Check sheet for the modelled part. Datum: model origin and axes. Units: mm. Face numbers are marked on the shaded views. A direction names the side the tool comes from. Round coordinates to 2 decimals unless told otherwise and drop trailing zeros. Loops run counter-clockwise (first coordinate to the right, second up) from the corner with the lowest first, then second, coordinate; pieces in that order, holes last. Notation, with made-up numbers: (54.25, 9) -> (72.25, 9) arc R27 cw to (72.25, 30) -> close; hole circle Ø6 at (88.25, -23). An arc over 180 degrees is marked (long way). Use one line per item in the form item = value. Start each with the question number.
(1) Sectioned sample at A-A (z = 7). Record the cut outline in (x, y).
(2) Sectioned sample at B-B (y = -9). Record the cut outline in (x, z).
(3) Sectioned sample at D-D (x = 1). State how many separate pieces and enclosed holes the cut face has, and give its area (3 significant figures).
(4) Material ranges on probe 1 along Z at (x, y) = (5, 6); probe 2 along Z at (x, y) = (4.75, -1); probe 3 along X at (y, z) = (-10.5, -8.5), recorded low to high. Write a range as [from, to].
(5) Set-up check for the marked faces 5 and 6: record each of +Z, -Z, +X, -X, +Y, -Y from which the full face is reachable in a straight line by a thin tool's end or side.
(6) Sectioned sample at C-C (z = -5). Record the cut outline in (x, y).
(7) Draft check along Y on the marked faces 1, 2, 3 and 4. Enter one of: released by +Y, released by -Y, zero draft, split by the parting line, or undercut.
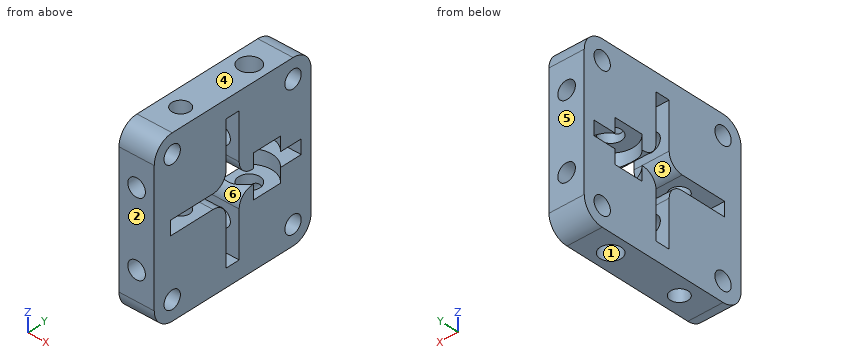
Autodesk Inventor part; units mm, degrees
ref_plane "YZ Plane" through (0, 0, 0) normal (1, 0, 0) x (0, 1, 0)
ref_plane "XZ Plane" through (0, 0, 0) normal (0, 1, 0) x (-1, 0, 0)
ref_plane "XY Plane" through (0, 0, 0) normal (0, 0, 1) x (1, 0, 0)
sketch "Sketch1" plane through (0, 0, 0) normal (1, 0, 0) x (0, 1, 0)
  circle A0 centre (0, 0) radius 2.8284
  line L0 (0, 0) -> (-2.8284, 0)
  line L1 (-2.8284, 0) -> (-2.8284, -2.8284)
  line L2 (-2.8284, -2.8284) -> (0, -2.8284)
  line L3 (0, -2.8284) -> (0, 0)
  line L4 (0, 0) -> (-2.8284, -2.8284)
  line L5 (2, 2) -> (-2, 2)
  line L6 (-2, 2) -> (-2, -2)
  line L7 (-2, -2) -> (2, -2)
  line L8 (2, -2) -> (2, 2)
  line L9 (2, 2) -> (-2, -2) construction
  line L10 (-2, 2) -> (2, -2) construction
  line L11 (2, 2) -> (-2, 2)
  line L12 (-2, 2) -> (-2, 4)
  line L13 (-2, 4) -> (2, 4)
  line L14 (2, 4) -> (2, 2)
  line L15 (0, 4) -> (0, 19)
  line L16 (-2, 2) -> (-4, 2)
  line L17 (-4, 2) -> (-4, -2)
  line L18 (-4, -2) -> (-2, -2)
  line L19 (-4, 0) -> (-19, 0)
  line L20 (19, -19) -> (19, 19)
  line L21 (19, 19) -> (-19, 19)
  line L22 (-19, 19) -> (-19, -19)
  line L23 (-19, -19) -> (19, -19)
  line L24 (19, -19) -> (-19, 19) construction
  line L25 (19, 19) -> (-19, -19) construction
  line L26 (0, 19) -> (0, 24)
  line L27 (-19, 0) -> (-24, 0)
  line L28 (24, -24) -> (24, 24)
  line L29 (24, 24) -> (-24, 24)
  line L30 (-24, 24) -> (-24, -24)
  line L31 (-24, -24) -> (24, -24)
  line L32 (24, -24) -> (-24, 24) construction
  line L33 (24, 24) -> (-24, -24) construction
  line L34 (-2, 2) -> (-19, 2)
  line L35 (-19, -2) -> (-2, -2)
  line L36 (-2, -2) -> (-2, 2)
  line L37 (-2, -2) -> (-19, -2)
  line L38 (-19, -2) -> (-19, -19)
  line L39 (-19, -19) -> (-2, -19)
  line L40 (-2, -19) -> (-2, -2)
  line L41 (2, -2) -> (19, -2)
  line L42 (19, -2) -> (19, -19)
  line L43 (19, -19) -> (2, -19)
  line L44 (2, -19) -> (2, -2)
  line L45 (2, 2) -> (19, 2)
  line L46 (19, 2) -> (19, 19)
  line L47 (19, 19) -> (2, 19)
  line L48 (2, 19) -> (2, 2)
  line L49 (-2, 2) -> (-19, 2)
  line L50 (-19, 2) -> (-19, 19)
  line L51 (-19, 19) -> (-2, 19)
  line L52 (-2, 19) -> (-2, 2)
  point P0 (-2, 19)
  point P1 (2, 4)
  point P2 (2, -19)
  point P3 (-2, -19)
  dimension "d0" = 4
  dimension "d1" = 2
  dimension "d5" = 15
  dimension "d6" = 2
  dimension "d7" = 15
  dimension "d8" = 2
  dimension "d9" = 0
  dimension "d10" = 5
  dimension "d11" = 5
  dimension "d12" = 15
  dimension "d13" = 22.6716
  dimension "d14" = 20
  dimension "d15" = 29.7321
extrude "Extrusion1" add sketch "Sketch1" along normal blind 10 contours L14 L48 L21 L20 L45 | L41 L20 L23 L44 | L16 L34 L22 L21 L52 L12 | L20 L21 L26 L29 L28 L31 L30 L27 L22 L23 | L40 L2 L4 | L4 L1 L18 | L40 L23 L22 L35 L18 L1 L2 | L21 L22 L27 L30 L29 L26
sketch "Sketch2" plane through (0, 24, 24) normal (0, 1, 0) x (1, 0, 0)
  line L0 (10, 0) -> (0, 0)
  line L1 (0, 0) -> (0, 48)
  line L2 (0, 48) -> (10, 48)
  line L3 (10, 48) -> (10, 0)
  line L4 (0, 48) -> (10, 48)
  line L5 (0, 48) -> (0, 34.5)
  line L6 (0, 34.5) -> (5, 34.5)
  circle A0 centre (5, 34.5) radius 2.5
  line L7 (0, 0) -> (0, 13.5)
  line L8 (0, 22) -> (0, 5)
  line L9 (0, 13.5) -> (5, 13.5)
  circle A1 centre (5, 13.5) radius 2.5
  point P0 (0, 24)
  dimension "d18" = 13.5
  dimension "d19" = 5
  dimension "d20" = 5
  dimension "d21" = 13.5
  dimension "d22" = 5
  dimension "d23" = 5
extrude "Extrusion2" cut sketch "Sketch2" against normal through all contours A0 | A1
sketch "Sketch3" plane through (0, -24, -24) normal (0, 0, -1) x (-1, 0, 0)
  line L0 (0, 0) -> (-10, 0)
  line L1 (0, 0) -> (0, 13.5)
  line L2 (0, 22) -> (0, 5)
  line L3 (0, 48) -> (-10, 48)
  line L4 (0, 48) -> (0, 34.5)
  line L5 (0, 0) -> (0, 48)
  line L6 (0, 34.5) -> (-5, 34.5)
  line L7 (0, 13.5) -> (-5, 13.5)
  circle A0 centre (-5, 13.5) radius 2.5
  circle A1 centre (-5, 34.5) radius 2.5
  point P0 (0, 24)
  dimension "d26" = 13.5
  dimension "d27" = 13.5
  dimension "d28" = 5
  dimension "d29" = 5
  dimension "d30" = 5
  dimension "d31" = 5
extrude "Extrusion3" cut sketch "Sketch3" against normal through all
fillet "Fillet1" radius 4 4 edges at (5, -2, 2) (5, 2, 2) (5, 2, -2) (5, -2, -2)
sketch "Sketch4" plane through (10, 0, 0) normal (1, 0, 0) x (0, 0, -1)
  line L0 (24, 24) -> (-24, 24)
  line L1 (24, 24) -> (18.5, 24)
  line L2 (18.5, 24) -> (18.5, 18.5)
  line L3 (18.5, 18.5) -> (24, 18.5)
  line L4 (24, 18.5) -> (24, 24)
  circle A0 centre (18.5, 18.5) radius 2.5
  circle A1 centre (18.5, 18.5) radius 5.5
  circle A2 centre (-18.5, 18.5) radius 5.5
  circle A3 centre (-18.5, 18.5) radius 2.5
  line L5 (-18.5, 24) -> (-24, 24)
  line L6 (-24, 24) -> (-24, 18.5)
  circle A4 centre (-18.5, -18.5) radius 5.5
  circle A5 centre (-18.5, -18.5) radius 2.5
  line L7 (-24, -18.5) -> (-24, -24)
  line L8 (-24, -24) -> (-18.5, -24)
  circle A6 centre (18.5, -18.5) radius 5.5
  circle A7 centre (18.5, -18.5) radius 2.5
  line L9 (18.5, -24) -> (24, -24)
  line L10 (24, -24) -> (24, -18.5)
  point P0 (0, 0)
  point P1 (-18.5, 24)
  dimension "d35" = 5.5
  dimension "d36" = 5.5
  dimension "d37" = 5
  dimension "d40" = 360
extrude "Extrusion4" cut sketch "Sketch4" against normal through all contours L4 A1 L0 | A2 L6 L0 | A0 L3 L2 | L2 L3 A0 | A3 | A4 L8 L7 | A5 | L10 L9 A6 | A7
sketch "Sketch5" plane through (0, -18.5, 24) normal (0, 0, 1) x (1, 0, 0)
  circle A0 centre (5, 29) radius 2.5
  circle A1 centre (5, 29) radius 3
  point P0 (0, 18.5)
  dimension "d44" = 6
extrude "Extrusion5" cut sketch "Sketch5" against normal through all contours A0 | A1
sketch "Sketch6" plane through (0, 19, -2) normal (0, 0, 1) x (1, 0, 0)
  circle A0 centre (5, -8.5) radius 6.5
  point P0 (0, -19)
extrude "Extrusion6" cut sketch "Sketch6" against normal blind 4
sketch "Sketch7" plane through (10, 19, 2) normal (0, 0, -1) x (-1, 0, 0)
  circle A0 centre (5, -8.5) radius 6.5
  point P0 (10, -19)
extrude "Extrusion7" cut sketch "Sketch7" against normal blind 4
sketch "Sketch8" plane through (10, 0, 0) normal (1, 0, 0) x (0, 0, -1)
  line L0 (-2, 14.6533) -> (-2, 19)
  line L1 (-2, 19) -> (2, 19)
  line L2 (2, 19) -> (2, 21)
  line L3 (2, 21) -> (-2, 21)
  line L4 (-2, 21) -> (-2, 19)
  point P0 (0, 0)
  dimension "d51" = 2
extrude "Extrusion8" cut sketch "Sketch8" against normal through all
properties part number "guidance_block" material "PET Plastic"
Checks:
q1.outline = (0, -24) -> (10, -24) -> (10, -2) -> (0, -2) -> close; (0, 2) -> (10, 2) -> (10, 24) -> (0, 24) -> close; hole circle Ø6 at (5, 10.5); hole circle Ø5 at (5, -10.5)
q2.outline = (0, -24) -> (3, -24) -> (3, -12) arc R2.5 cw to (3, -9) -> (3, -2) -> (0, -2) -> close; (0, 2) -> (3, 2) -> (3, 9) arc R2.5 cw to (3, 12) -> (3, 24) -> (0, 24) -> close; (7, -24) -> (10, -24) -> (10, -2) -> (7, -2) -> (7, -9) arc R2.5 cw to (7, -12) -> close; (7, 2) -> (10, 2) -> (10, 24) -> (7, 24) -> (7, 12) arc R2.5 cw to (7, 9) -> close
q3.separate_pieces = 1
q3.enclosed_holes = 5
q3.area = 1,810 mm2
q4.probe_1 = [-24, -13], [-8, -6], [6, 8], [13, 24]
q4.probe_2 = [-24, -19], [19, 24]
q4.probe_3 = [0, 2.5], [7.5, 10]
q5.face_5 = +Z, -Z, +X, -X, +Y
q5.face_6 = +X, -X
q6.outline = (0, -24) -> (10, -24) -> (10, -2.13) -> (0, -2.13) -> close; (0, 2.13) -> (10, 2.13) -> (10, 6.35) arc R6.5 cw to (0, 6.35) -> close; (0, 14.65) arc R6.5 cw to (10, 14.65) -> (10, 24) -> (0, 24) -> close; hole circle Ø5 at (5, -10.5)
q7.face_1 = undercut
q7.face_2 = released by -Y
q7.face_3 = undercut
q7.face_4 = zero draft
